from build123d import *

# Parameters (mm, degrees)
PAD_DEPTH            = 6.5
POCKET_DEPTH         = 6
SKETCH002_R          = 13.5
POCKET001_DEPTH      = 1
SKETCH003_W          = 5.4
SKETCH003_H          = 6.5
PAD001_DEPTH         = 4.5
POCKET002_DEPTH      = 10
SKETCH010_W          = 3.95
SKETCH010_H          = 6.5
PAD002_DEPTH         = 4.5
POCKET005_DEPTH      = 10
SKETCH014_R          = 20.45
SKETCH014_R_2        = 19.5
POCKET008_DEPTH      = 0.3
SKETCH015_R          = 2.2
SKETCH015_R_2        = 0.975
PAD003_DEPTH         = 2
POCKET009_DEPTH      = 4
POCKET010_DEPTH      = 4
PAD004_DEPTH         = 4
SKETCH019_R          = 0.6
POCKET011_DEPTH      = 2
SKETCH020_R          = 0.6
POCKET012_DEPTH      = 2
POCKET013_DEPTH      = 12.151
POCKET013_DEPTH_BACK = 36.251


with BuildPart() as part:
    # Sketch → Pad (new body)
    with BuildSketch(Plane.XY):
        with BuildLine():
            Line((-22.5019915649, 16), (-22.5019915649, -16))
            Line((-22.5019915649, -16), (-16.2858834577, -17.9000000001))
            ThreePointArc((-16.2858834577, -17.9000000001), (0.2206895737, -24.1989937004), (16.6096357576, -17.5999999999))
            Line((16.6096357576, -17.5999999999), (24.9082802252, -17.45))
            Line((24.9082802252, 17.45), (24.9082802252, -17.45))
            Line((16.6096357576, 17.6), (24.9082802252, 17.45))
            ThreePointArc((16.6096357576, 17.6), (0.2206895736, 24.1989937004), (-16.2858834578, 17.9))
            Line((-22.5019915649, 16), (-16.2858834578, 17.9))
        make_face()
    extrude(amount=PAD_DEPTH)

    # Sketch001 → Pocket (cut)
    with BuildSketch(Plane.XY):
        with BuildLine():
            Line((-14.8539557021, 16.9), (-21.2122180433, 15.55))
            Line((-21.2122180433, 15.55), (-21.2122180433, -15.55))
            Line((-21.2122180433, -15.55), (-14.8539557021, -16.9))
            ThreePointArc((-14.8539557021, -16.9), (-0.0760301383, -22.4998715423), (14.739402973, -17))
            Line((14.739402973, -17), (23.6191552218, -16.4))
            Line((23.6191552218, 16.4), (23.6191552218, -16.4))
            Line((14.739402973, 17), (23.6191552218, 16.4))
            ThreePointArc((14.739402973, 17), (-0.0760301383, 22.4998715423), (-14.8539557021, 16.9))
        make_face()
    extrude(amount=POCKET_DEPTH, mode=Mode.SUBTRACT)

    # Sketch002 (on Face19 of Pocket) → Pocket001 (cut)
    with BuildSketch(Plane(origin=(0, 0, 6), x_dir=(1, 0, 0), z_dir=(0, 0, -1))):
        Circle(SKETCH002_R)
    extrude(amount=-POCKET001_DEPTH, mode=Mode.SUBTRACT)

    # Sketch003 (on Face7 of Pad) → Pad001 (join)
    with BuildSketch(Plane.YZ.offset(24.9082802252)):
        with Locations((-14.75, 3.25)):
            Rectangle(SKETCH003_W, SKETCH003_H)
        with Locations((14.75, 3.25)):
            Rectangle(SKETCH003_W, SKETCH003_H)
    extrude(amount=PAD001_DEPTH)

    # Sketch006 (on Face22 of Pad001) → Pocket002 (cut)
    with BuildSketch(Plane.XY.offset(6.5)):
        with BuildLine():
            ThreePointArc((24.9082802252, 17.45), (26.9423471239, 15.7065020586), (29.4082802252, 14.6594169811))
            Line((29.4082802252, 17.45), (29.4082802252, 14.6594169811))
            Line((29.4082802252, 17.45), (24.9082802252, 17.45))
        make_face()
        with BuildLine():
            ThreePointArc((29.4082802252, -14.6594169811), (26.9423471239, -15.7065020586), (24.9082802252, -17.45))
            Line((29.4082802252, -17.45), (24.9082802252, -17.45))
            Line((29.4082802252, -14.6594169811), (29.4082802252, -17.45))
        make_face()
    extrude(amount=-POCKET002_DEPTH, mode=Mode.SUBTRACT)

    # Sketch010 (on Face3 of Pad) → Pad002 (join)
    with BuildSketch(Plane(origin=(-22.5019915649, 0, 0), x_dir=(0, -1, 0), z_dir=(-1, 0, 0))):
        with Locations((-14.025, 3.25)):
            Rectangle(SKETCH010_W, SKETCH010_H)
        with Locations((14.025, 3.25)):
            Rectangle(SKETCH010_W, SKETCH010_H)
    extrude(amount=PAD002_DEPTH)

    # Sketch011 (on Face28 of Pad002) → Pocket005 (cut)
    with BuildSketch(Plane.XY.offset(6.5)):
        Polygon((-27.0019915649, 16), (-22.5019915649, 16), (-27.0019915649, 14.5), align=None)
        Polygon((-22.5019915649, -16), (-27.0019915649, -14.5), (-27.0019915649, -16), align=None)
    extrude(amount=-POCKET005_DEPTH, mode=Mode.SUBTRACT)

    # Sketch014 (on Face10 of Pad) → Pocket008 (cut)
    with BuildSketch(Plane.XY.offset(6.5)):
        Circle(SKETCH014_R)
        Circle(SKETCH014_R_2, mode=Mode.SUBTRACT)
    extrude(amount=-POCKET008_DEPTH, mode=Mode.SUBTRACT)

    # Sketch015 (on Face19 of Pocket) → Pad003 (join)
    with BuildSketch(Plane(origin=(0, 0, 6), x_dir=(1, 0, 0), z_dir=(0, 0, -1))):
        with Locations((-18.42, 13.32)):
            Circle(SKETCH015_R)
        with Locations((-18.42, 13.32)):
            Circle(SKETCH015_R_2, mode=Mode.SUBTRACT)
        with Locations((7.27, 18.56)):
            Circle(SKETCH015_R)
        with Locations((7.27, 18.56)):
            Circle(SKETCH015_R_2, mode=Mode.SUBTRACT)
        with Locations((5.37, -19.79)):
            Circle(SKETCH015_R)
        with Locations((5.37, -19.79)):
            Circle(SKETCH015_R_2, mode=Mode.SUBTRACT)
        with Locations((-18.42, -13.32)):
            Circle(SKETCH015_R)
        with Locations((-18.42, -13.32)):
            Circle(SKETCH015_R_2, mode=Mode.SUBTRACT)
    extrude(amount=PAD003_DEPTH)

    # Sketch016 → Pocket009 (cut)
    with BuildSketch(Plane(origin=(0, 0, 0), x_dir=(-1, 0, 0), z_dir=(0, 0, 1))):
        with BuildLine():
            Line((-5, 23.6778377391), (-5, 21.9374109685))
            ThreePointArc((5, 21.9374109685), (0, 22.5), (-5, 21.9374109685))
            Line((5, 23.6778377391), (5, 21.9374109685))
            ThreePointArc((5, 23.6778377391), (0, 24.2), (-5, 23.6778377391))
        make_face()
    extrude(amount=POCKET009_DEPTH, mode=Mode.SUBTRACT)

    # Sketch017 → Pocket010 (cut)
    with BuildSketch(Plane(origin=(0, 0, 0), x_dir=(-1, 0, 0), z_dir=(0, 0, 1))):
        with BuildLine():
            Line((-3.499984119, -22.2261132717), (-3.5, -23.9455632634))
            ThreePointArc((-3.5, -23.9455632634), (0, -24.2000019575), (3.5, -23.9455632634))
            Line((3.5000158811, -22.2261082701), (3.5, -23.9455632634))
            ThreePointArc((-3.499984119, -22.2261132717), (1.60767e-05, -22.5), (3.5000158811, -22.2261082701))
        make_face()
        with BuildLine():
            ThreePointArc((-13.9498796389, -17.6536358312), (-11.25, -19.4855715851), (-8.3135572795, -20.9077680626))
            Line((-8.3135572795, -20.9077680626), (-8.9416927184, -22.487466094))
            ThreePointArc((-15.0038705449, -18.987466094), (-12.1, -20.9578147716), (-8.9416927184, -22.487466094))
            Line((-13.9498796389, -17.6536358312), (-15.0038705449, -18.987466094))
        make_face()
        with BuildLine():
            ThreePointArc((8.3135572795, -20.9077680626), (11.25, -19.4855715851), (13.9498796389, -17.6536358312))
            Line((13.9498796389, -17.6536358312), (15.0038705449, -18.987466094))
            ThreePointArc((8.9416927184, -22.487466094), (12.1, -20.9578147716), (15.0038705449, -18.987466094))
            Line((8.3135572795, -20.9077680626), (8.9416927184, -22.487466094))
        make_face()
    extrude(amount=POCKET010_DEPTH, mode=Mode.SUBTRACT)

    # Sketch018 (on Face8 of Pocket005) → Pad004 (join)
    with BuildSketch(Plane(origin=(0, 0, 0), x_dir=(1, 0, 0), z_dir=(0, 0, -1))):
        Polygon((-27.0019915649, 14.5), (-27.0019915649, 12.05), (-22.5019915649, 12.05), (-22.5019915649, 16), align=None)
        Polygon((-27.0019915649, -12.05), (-22.5019915649, -12.05), (-22.5019915649, -16), (-27.0019915649, -14.5), align=None)
        with BuildLine():
            Line((24.9082802252, 17.45), (24.9082802252, 12.05))
            Line((29.4082802252, 12.05), (24.9082802252, 12.05))
            Line((29.4082802252, 14.6594169811), (29.4082802252, 12.05))
            ThreePointArc((24.9082802252, 17.45), (26.9423471239, 15.7065020586), (29.4082802252, 14.6594169811))
        make_face()
        with BuildLine():
            Line((24.9082802252, -12.05), (24.9082802252, -17.45))
            ThreePointArc((29.4082802252, -14.6594169811), (26.9423471239, -15.7065020586), (24.9082802252, -17.45))
            Line((29.4082802252, -12.05), (29.4082802252, -14.6594169811))
            Line((24.9082802252, -12.05), (29.4082802252, -12.05))
        make_face()
    extrude(amount=PAD004_DEPTH)

    # Sketch019 (on Face64 of Pad004) → Pocket011 (cut)
    with BuildSketch(Plane.XZ.offset(-12.05)):
        with Locations((28.1082802252, -2.7)):
            Circle(SKETCH019_R)
        with Locations((-25.7019915649, -2.7)):
            Circle(SKETCH019_R)
    extrude(amount=-POCKET011_DEPTH, mode=Mode.SUBTRACT)

    # Sketch020 (on Face50 of Pocket011) → Pocket012 (cut)
    with BuildSketch(Plane(origin=(0, -12.05, 0), x_dir=(-1, 0, 0), z_dir=(0, 1, 0))):
        with Locations((-28.1082802252, -2.7)):
            Circle(SKETCH020_R)
        with Locations((25.7019915649, -2.7)):
            Circle(SKETCH020_R)
    extrude(amount=-POCKET012_DEPTH, mode=Mode.SUBTRACT)

    # Sketch021 (on Face48 of Pocket012) → Pocket013 (cut, two sides)
    with BuildSketch(Plane.XZ.offset(-12.05)) as pocket013_sk:
        with BuildLine():
            ThreePointArc((29.4082802252, 0), (28.1735037783, 3.9528470752), (24.9082802252, 6.5))
            Line((24.9082802252, 6.5), (29.4082802252, 6.5))
            Line((29.4082802252, 6.5), (29.4082802252, 0))
        make_face()
        with BuildLine():
            ThreePointArc((24.9082802252, -1.478433716), (25.9291187082, -3.0916708473), (27.6082802252, -4))
            Line((24.9082802252, -4), (27.6082802252, -4))
            Line((24.9082802252, -1.478433716), (24.9082802252, -4))
        make_face()
        with BuildLine():
            ThreePointArc((-22.5019915649, 6.5), (-25.767215118, 3.9528470752), (-27.0019915649, 0))
            Line((-27.0019915649, 6.5), (-27.0019915649, 0))
            Line((-22.5019915649, 6.5), (-27.0019915649, 6.5))
        make_face()
        with BuildLine():
            ThreePointArc((-25.3019915649, -4), (-23.3759624024, -3.1260291625), (-22.5019915649, -1.2))
            Line((-22.5019915649, -1.2), (-22.5019915649, -4))
            Line((-22.5019915649, -4), (-25.3019915649, -4))
        make_face()
    extrude(amount=-POCKET013_DEPTH, mode=Mode.SUBTRACT)
    extrude(pocket013_sk.sketch, amount=POCKET013_DEPTH_BACK, mode=Mode.SUBTRACT)


solid = part.part
Work out the finished part from the listing and answer in its coordinate system (mm). A direction names the side the tool comes from. Give positions to 0.01 mm unless a question says otherwise; leave off trailing zeros. Loops run counter-clockwise (first coordinate to the right, second up) from the corner with the lowest first, then second, coordinate; pieces in that order, holes last. Notation, with made-up numbers: (60.5, -15) -> (107.5, -15) arc R36 ccw to (107.5, 19) -> close; hole circle Ø7 at (2.25, 59). An arc over 180 degrees is marked (long way). Use a Markdown table: item, result. Add a question column.
1. Determine the mould class of faces 6 (the flat face through (-25, -12.05, 0)), 7 (the flat face through (-26, -14.05, -3)), 8 (the flat face through (28, 14.05, -3)), 9 (the flat face through (28, 14, -4)) for opening direction Z: released by +Z, released by -Z, zero draft, split by the parting line, or undercut.
2. Section D-D on x = 21.5 is taken. Determine the outline of the cut face in (y, z), and give its area (3 significant figures).
3. Section B-B on y = 0 is taken. Determine the outline of the cut face in (x, z), and give its area (3 significant figures).
4. For faces 1 (the cylindrical face through (-25.733, 13.558, 4.001)), 2 (the flat face through (14.47, 18.31, 1.97)), 3 (the flat face through (7, -19, 6)), 4 (the cylindrical face through (27.63, 13.51, 4.64)), 5 (the cylindrical face through (-14.37, 13.18, 6.35)), determine the directions among +Z, -Z, +X, -X, +Y, -Y from which every point of the face is accessible in a straight line to the end or side of a thin tool.
5. Section C-C on z = 5.25 is taken. State how many separate pieces and enclosed holes the cut face has, and give its area (3 significant figures).
6. Section A-A on x = 0 is taken. Determine the outline of the cut face in (y, z), and give its area (3 significant figures).
7. Find the intervals of material crossed by probe 1 along X at (y, z) = (0, 6.1); probe 2 along X at (y, z) = (-8, 2.25); probe 3 along Y at (x, z) = (-18.42, 4.75) (3 decimals), in increasing order.
8. Flat-ended cylindrical pins translate along their axes: pin 1 Ø1.1 at (x, z) = (-25.7, -2.7) entering from +Y; pin 2 Ø1.5 at (x, y) = (-6, 23) entering from -Z; pin 3 Ø1.8 at (y, z) = (7.5, 3) entering from -X; pin 4 Ø24.5 at (x, y) = (0, 0) entering from -Z. Find the tip coordinate at first contact, or state that the pin passes through.
Results below:
| question | item | result |
|---|---|---|
| 1 | face 6 | zero draft |
| 1 | face 7 | undercut |
| 1 | face 8 | undercut |
| 1 | face 9 | released by -Z |
| 2 | outline | (-17.51, 0) -> (-16.54, 0) -> (-16.54, 6) -> (16.54, 6) -> (16.54, 0) -> (17.51, 0) -> (17.51, 6.5) -> (-17.51, 6.5) -> close |
| 2 | area | 29.1 mm^2 |
| 3 | outline | (-22.5, 0) -> (-21.21, 0) -> (-21.21, 6) -> (-13.5, 6) -> (-13.5, 6.5) -> (-19.5, 6.5) -> (-19.5, 6.2) -> (-20.45, 6.2) -> (-20.45, 6.5) -> (-22.5, 6.5) -> close; (13.5, 6) -> (23.62, 6) -> (23.62, 0) -> (24.91, 0) -> (24.91, 6.5) -> (20.45, 6.5) -> (20.45, 6.2) -> (19.5, 6.2) -> (19.5, 6.5) -> (13.5, 6.5) -> close |
| 3 | area | 25.1 mm^2 |
| 4 | face 1 | +Z, -X, +Y, -Y |
| 4 | face 2 | -Z, +Y |
| 4 | face 3 | -Z |
| 4 | face 4 | +Z, +X, +Y, -Y |
| 4 | face 5 | +Z |
| 5 | separate pieces | 4 |
| 5 | enclosed holes | 5 |
| 5 | area | 312 mm^2 |
| 6 | outline | (-24.2, 4) -> (-22.5, 4) -> (-22.5, 6) -> (-13.5, 6) -> (-13.5, 6.5) -> (-19.5, 6.5) -> (-19.5, 6.2) -> (-20.45, 6.2) -> (-20.45, 6.5) -> (-24.2, 6.5) -> close; (13.5, 6) -> (22.5, 6) -> (22.5, 4) -> (24.2, 4) -> (24.2, 6.5) -> (20.45, 6.5) -> (20.45, 6.2) -> (19.5, 6.2) -> (19.5, 6.5) -> (13.5, 6.5) -> close |
| 6 | area | 16.9 mm^2 |
| 7 | probe 1 | x = -22.5 to -13.5, 13.5 to 24.91 |
| 7 | probe 2 | x = -22.5 to -21.21, 23.62 to 24.91 |
| 7 | probe 3 | y = -17.248 to -16.143, -15.52 to -14.295, -12.345 to -11.12, 11.12 to 12.345, 14.295 to 15.52, 16.143 to 17.248 |
| 8 | pin 1 | stops at y = 15.12 |
| 8 | pin 2 | stops at z = 0 |
| 8 | pin 3 | stops at x = -22.5 |
| 8 | pin 4 | passes through |
